```python
from build123d import *

# Parameters (mm, degrees)
F0_R     = 10
F1_DEPTH = 20
F2_W     = 20
F2_H     = 40
F3_DEPTH = 20
F4_W     = 20
F4_H     = 20
F5_DEPTH = 10


with BuildPart() as f1:
    # F0 (on Front) → F1 (new body)
    with BuildSketch(Plane.XZ):
        with BuildLine():
            Line((-40, 40), (-40, 0))
            Line((-40, 0), (0, 0))
            ThreePointArc((0, 0), (19.968011, 20), (0, 40))
            Line((0, 40), (-40, 40))
        make_face()
        with Locations((-0.032014, 20)):
            Circle(F0_R, mode=Mode.SUBTRACT)
    extrude(amount=F1_DEPTH)

    # F2 (on face) → F3 (join)
    with BuildSketch(Plane.XZ.offset(20)):
        with Locations((-30, 20)):
            Rectangle(F2_W, F2_H)
    extrude(amount=F3_DEPTH)

    # F4 (on face) → F5 (cut)
    with BuildSketch(Plane.XZ.offset(40)):
        with Locations((-30, 20)):
            Rectangle(F4_W, F4_H)
    extrude(amount=-F5_DEPTH, mode=Mode.SUBTRACT)


solid = f1.part
```
The listing builds one solid part. Answer for the finished solid, in the listing's coordinates (mm). A direction names the side the tool comes from. Round coordinates to 2 decimals unless told otherwise and drop trailing zeros. Loops run counter-clockwise (first coordinate to the right, second up) from the corner with the lowest first, then second, coordinate; pieces in that order, holes last. Notation, with made-up numbers: (7.25, 34) - (21.25, 34) arc R7 ccw to (21.25, 38) - close; hole circle Ø1 at (10, 88.5). An arc over 180 degrees is marked (long way). Use one line per item in the form item = value. Start each with the question number.
1. Consider line 1 (Z direction, x = -34.5, y = -36); line 2 (Y direction, x = 17.5, z = 27.5); line 3 (X direction, y = -14.5, z = 28). Determine where each line is inside the solid, lowest interval first. Write a range as [from, to].
2. The part is cut by section B-B on y = -36. Determine the outline of the cut face in (x, z), then the cut area to 3 significant figures.
3. The part is cut by section D-D on x = 7. Determine the outline of the cut face in (y, z), then the cut area to 3 significant figures.
4. A tool of negligible diameter and unlimited length cuts with its end or side. For faces 1 (the face through (-30, -40, 5)), 2 (the face through (-30, -35, 10)), 3 (the face through (-20, -28, 20)), from which of +Z, -Z, +X, -X, +Y, -Y can it reach the whole face along a straight path? Write none if from no direction.
5. The part is cut by section A-A on z = 20. Determine the outline of the cut face in (x, y), then the cut area to 3 significant figures.
6. For a pull along Z with two mould halves and no side action, classify faces 4 (the face through (-30, -30, 20)), 5 (the face through (-17, 0, 20)), 6 (the face through (-25, -15, 0)), 7 (the face through (-25, -15, 40)) as pulls with the +Z half, pulls with the -Z half, needs draft (parallel to the pull), parting line crosses it, or undercut.
7. Given pin 1 Ø1.5 at (x, y) = (9.5, -5) entering from -Z; pin 2 Ø4 at (x, z) = (-32, 27.5) entering from -Y, each flat-ended and moving along its own axis, determine where each tip first touches the part or whether it passes through.
8. The part is cut by section C-C on y = -6. Determine the outline of the cut face in (x, z).
Geometry check:
q1.line_1 = [0, 10], [30, 40]
q1.line_2 = [-20, 0]
q1.line_3 = [-40, -6.03], [5.97, 18.3]
q2.outline = (-40, 0) - (-20, 0) - (-20, 10) - (-40, 10) - close; (-40, 30) - (-20, 30) - (-20, 40) - (-40, 40) - close
q2.area = 400 mm^2
q3.outline = (-20, 1.28) - (0, 1.28) - (0, 12.89) - (-20, 12.89) - close; (-20, 27.11) - (0, 27.11) - (0, 38.72) - (-20, 38.72) - close
q3.area = 465 mm^2
q4.face_1 = +Z, -Z, +X, -X, -Y
q4.face_2 = +X, -X, -Y
q4.face_3 = +Z, -Z, +X, -Y
q5.outline = (-40, -30) - (-20, -30) - (-20, -20) - (-10.03, -20) - (-10.03, 0) - (-40, 0) - close; (9.97, -20) - (19.97, -20) - (19.97, 0) - (9.97, 0) - close
q5.area = 999 mm^2
q6.face_4 = undercut
q6.face_5 = needs draft
q6.face_6 = pulls with the -Z half
q6.face_7 = pulls with the +Z half
q7.pin_1 = 2.03
q7.pin_2 = -30
q8.outline = (-40, 0) - (0, 0) arc R20 ccw to (0, 40) - (-40, 40) - close; hole circle Ø20 at (-0.03, 20)
